Check sheet for the modelled part. Datum: model origin and axes. Units: mm. Face numbers are marked on the shaded views. A direction names the side the tool comes from. Round coordinates to 2 decimals unless told otherwise and drop trailing zeros. Loops run counter-clockwise (first coordinate to the right, second up) from the corner with the lowest first, then second, coordinate; pieces in that order, holes last. Notation, with made-up numbers: M 61,-28 L 104,-28 A37 cw 104,8 Z; hole C 87,4.5 d8. An arc over 180 degrees is marked long. Write item = value, one per line. Start each with the question number.
(1) Cross-section at B-B on x = -4.25. Record the boundary of the cut face in (y, z) (3 decimals).
(2) Set-up check for the marked faces 5 and 6: record each of +Z, -Z, +X, -X, +Y, -Y from which the full face is reachable in a straight line by a thin tool's end or side.
(3) Scan lines: L1, parallel to Y at x = 5, z = 8.25; L2, parallel to X at y = -1.5, z = 5; L3, parallel to X at y = 7, z = 8.25. Record each from-to range of solid material in increasing order. Write a range as from..to.
(4) Cross-section at C-C on y = 8.5. Record the boundary of the cut face in (x, z) (3 decimals).
(5) Mould release check, pull along Y, two halves, no side actions. Record for the marked faces 1, 2, 3 and 4: pulls with the +Y half, pulls with the -Y half, needs draft (parallel to the pull), parting line crosses it, or undercut.
(6) Cross-section at D-D on y = 3.5. Record the boundary of the cut face in (x, z) (3 decimals).
(7) Go/stop test with flat-tipped pins: P1, Ø2, axis at x = 8.5, z = 2.5, coming from the +Y side; P2, Ø3, axis at x = 0, y = 5, coming from the +Z side; P3, Ø3, axis at x = 13.5, z = 2, coming from the +Y side; P4, Ø3, axis at y = 6, z = 4, coming from the +X side. Record where each tip stops, or that it passes through.
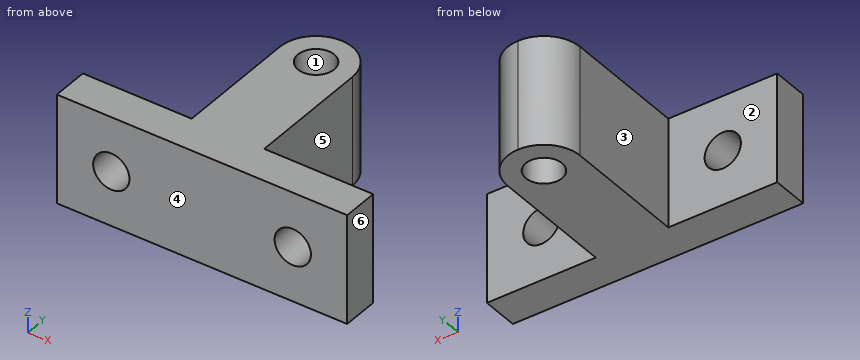
from build123d import *

# Parameters (mm, degrees)
F0_R     = 1.5875
F1_DEPTH = 9.525
F3_D     = 3.175
F5_D     = 3.175


# Not quite as in the source:
# - a length typed as a fraction of an inch, garbled in the dataset ("3 / 203.2 mm" for 3/8 in), is restored


with BuildPart() as f1:
    # F0 (on Top) → F1 (new body)
    with BuildSketch(Plane.XY):
        with BuildLine():
            Line((1.6785456881, 9.5886874095), (1.6785456881, -1.2063125905))
            Line((1.6785456881, -1.2063125905), (8.0285456881, -1.2063125905))
            Line((8.0285456881, -1.2063125905), (8.0285456881, 9.5886874095))
            ThreePointArc((8.0285456881, 9.5886874095), (7.0986097184, 11.8337514397), (4.8535456881, 12.7636874095))
            ThreePointArc((4.8535456881, 12.7636874095), (2.6084816578, 11.8337514397), (1.6785456881, 9.5886874095))
        make_face()
        with Locations((4.8535456881, 9.5886874095)):
            Circle(F0_R, mode=Mode.SUBTRACT)
        Polygon((-7.8464543119, -1.2063125905), (-7.8464543119, -4.3813125905), (17.5535456881, -4.3813125905), (17.5535456881, -1.2063125905), (8.0285456881, -1.2063125905), (1.6785456881, -1.2063125905), align=None)
    extrude(amount=F1_DEPTH)

    # F3 (through all)
    with Locations(Plane(origin=(0, -1.2063125905, 0), x_dir=(-1, 0, 0), z_dir=(0, 1, 0))):
        with Locations((-12.7910456881, 4.7625)):
            Hole(F3_D / 2)

    # F5 (through all)
    with Locations(Plane(origin=(0, -1.2063125905, 0), x_dir=(-1, 0, 0), z_dir=(0, 1, 0))):
        with Locations((3.0839543119, 4.7625)):
            Hole(F5_D / 2)


solid = f1.part
Result:
q1.outline = M -4.381,0 L -1.206,0 L -1.206,3.685 L -4.381,3.685 Z; M -4.381,5.84 L -1.206,5.84 L -1.206,9.525 L -4.381,9.525 Z
q2.face_5 = +Z, -Z, +X, +Y
q2.face_6 = +Z, -Z, +X, +Y, -Y
q3.L1 = -4.38..8.01, 11.17..12.76
q3.L2 = -7.85..-4.65, -1.51..11.22, 14.36..17.55
q3.L3 = 1.68..8.03
q4.outline = M 1.679,0 L 3.698,0 L 3.698,9.525 L 1.679,9.525 Z; M 6.009,0 L 8.029,0 L 8.029,9.525 L 6.009,9.525 Z
q5.face_1 = undercut
q5.face_2 = pulls with the +Y half
q5.face_3 = needs draft
q5.face_4 = pulls with the -Y half
q6.outline = M 1.679,0 L 8.029,0 L 8.029,9.525 L 1.679,9.525 Z
q7.P1 = 11.34
q7.P2 = through
q7.P3 = -1.21
q7.P4 = 8.03
